Geometry: final body of the model. Coordinates: model frame, mm. A direction names the side the tool comes from. Give positions to 0.01 mm unless a question says otherwise; leave off trailing zeros. Write each loop counter-clockwise with the first axis right and the second up, starting at its lowest first coordinate (ties: lowest second). Pieces come first, ordered by that corner, then holes.
Q1. Cut plane A-A on z = 11. Return the cut outline in (x, y).
Q2. Cut plane D-D on x = 69.5. Return the cut outline in (y, z).
Q3. Draft query along Y for faces 4 (the face through (20, 20, 10)), 5 (the face through (40.46, 0.6, 9.43)), 6 (the face through (12.504, 20.253, 17.395)), 7 (the face through (60, 20, 10)). Return one class per face: pulls with the +Y half, pulls with the -Y half, needs draft (parallel to the pull), parting line crosses it, or undercut.
Q4. Pin query (flat end, axial travel): pin 1 (12 mm diameter, centred on x = 46.5, z = 17, fed in from -Y); pin 2 (1 mm diameter, centred on x = 13, y = 32, fed in from +Z); pin 3 (4 mm diameter, centred on x = 19.5, z = 15.5, fed in from -Y). Return the tip coordinate at first contact, or that it passes through.
Q5. Cut plane B-B on y = 20. Return the cut outline in (x, z), plus the area to 3 significant figures.
Q6. Cut plane C-C on x = 53. Return the cut outline in (y, z).
Q7. Reachability of faces 1 (the face through (40, 15, 18)), 2 (the face through (40, 25, 18)), 3 (the face through (39, 20, 0)) from +Z, -Z, +X, -X, +Y, -Y: full face, straight path, thin tool, end or side. Return the list, or none.
Q8. Line query: L1, parallel to Y at x = 20, z = 20.5; L2, parallel to Z at x = 7.5, y = 37.5; L3, parallel to Y at x = 36, z = 18. Output: solid intervals per line, ascending.
```python
from build123d import *

# Parameters (mm, degrees)
BOSS_EXTRUDE1_DEPTH = 10
FILLET1_R           = 2
FILLET2_R           = 2
SKETCH2_R           = 7.5
BOSS_EXTRUDE3_DEPTH = 15
SKETCH3_R           = 5
CUT_EXTRUDE1_DEPTH  = 15
SKETCH4_R           = 5
CUT_EXTRUDE2_DEPTH  = 15
RIB1_REACH          = 94.871
SKETCH5_WALLS_W     = 202.74175621
SKETCH5_WALLS_H     = 10


with BuildPart() as part:
    # Sketch1 → Boss-Extrude1 (new body)
    with BuildSketch(Plane.XY):
        with BuildLine():
            Line((7, 0), (73, 0))
            ThreePointArc((73, 0), (77.949747468, 2.050252532), (80, 7))
            Line((80, 7), (80, 33))
            ThreePointArc((80, 33), (77.949747468, 37.949747468), (73, 40))
            Line((73, 40), (7, 40))
            ThreePointArc((7, 40), (2.050252532, 37.949747468), (0, 33))
            Line((0, 33), (0, 7))
            ThreePointArc((0, 7), (2.050252532, 2.050252532), (7, 0))
        make_face()
    extrude(amount=BOSS_EXTRUDE1_DEPTH)

    # Fillet1
    fillet1_edges = [part.edges().sort_by_distance(p)[0] for p in [
        (40, 40, 0),
        (2.050252532, 37.949747468, 0),
        (0, 20, 0),
        (2.050252532, 2.050252532, 0),
        (40, 0, 0),
        (77.949747468, 2.050252532, 0),
        (80, 20, 0),
        (77.949747468, 37.949747468, 0),
    ]]
    fillet(fillet1_edges, radius=FILLET1_R)

    # Fillet2
    fillet2_edges = [part.edges().sort_by_distance(p)[0] for p in [
        (2.050252532, 37.949747468, 10),
        (40, 40, 10),
        (77.949747468, 37.949747468, 10),
        (80, 20, 10),
        (77.949747468, 2.050252532, 10),
        (40, 0, 10),
        (2.050252532, 2.050252532, 10),
        (0, 20, 10),
    ]]
    fillet(fillet2_edges, radius=FILLET2_R)

    # Sketch2 → Boss-Extrude3 (add)
    with BuildSketch(Plane.XY.offset(10)):
        with Locations(Location((20, 20, 0), (0, 0, 180))):
            Circle(SKETCH2_R)
        with Locations(Location((60, 20, 0), (0, 0, 180))):
            Circle(SKETCH2_R)
    extrude(amount=BOSS_EXTRUDE3_DEPTH)

    # Sketch3 → Cut-Extrude1 (cut)
    with BuildSketch(Plane.XY.offset(25)):
        with Locations((20, 20)):
            Circle(SKETCH3_R)
    extrude(amount=-CUT_EXTRUDE1_DEPTH, mode=Mode.SUBTRACT)

    # Sketch4 → Cut-Extrude2 (cut)
    with BuildSketch(Plane.XY.offset(25)):
        with Locations((60, 20)):
            Circle(SKETCH4_R)
    extrude(amount=-CUT_EXTRUDE2_DEPTH, mode=Mode.SUBTRACT)

    # Sketch5 walls → Rib1 (add, up to next)
    with BuildSketch(Plane.XY.offset(25), mode=Mode.PRIVATE) as rib1_sk1:
        with Locations((40.936137708, 20)):
            Rectangle(SKETCH5_WALLS_W, SKETCH5_WALLS_H)
    rib1_tool1 = extrude(rib1_sk1.sketch, amount=-RIB1_REACH, mode=Mode.PRIVATE) - part.part
    add(rib1_tool1.solids().sort_by_distance((40.936137708, 20, 25))[0])


solid = part.part
```
Data:
1. outline: (25.59, 15) - (54.41, 15) arc R7.5 ccw (long way) to (54.41, 25) - (25.59, 25) arc R7.5 ccw (long way) to start; hole circle Ø10 at (20, 20); hole circle Ø10 at (60, 20)
2. outline: (0, 2) arc R2 ccw to (2, 0) - (38, 0) arc R2 ccw to (40, 2) - (40, 8) arc R2 ccw to (38, 10) - (2, 10) arc R2 ccw to (0, 8) - close
3. face 4: undercut
3. face 5: pulls with the -Y half
3. face 6: parting line crosses it
3. face 7: undercut
4. pin 1: stops at y = 15
4. pin 2: stops at z = 10
4. pin 3: stops at y = 12.5
5. outline: (0, 2) arc R2 ccw to (2, 0) - (78, 0) arc R2 ccw to (80, 2) - (80, 8) arc R2 ccw to (78, 10) - (67.5, 10) - (67.5, 25) - (65, 25) - (65, 10) - (55, 10) - (55, 25) - (25, 25) - (25, 10) - (15, 10) - (15, 25) - (12.5, 25) - (12.5, 10) - (2, 10) arc R2 ccw to (0, 8) - close
5. area: 1,320 mm2
6. outline: (0, 2) arc R2 ccw to (2, 0) - (38, 0) arc R2 ccw to (40, 2) - (40, 8) arc R2 ccw to (38, 10) - (25, 10) - (25, 25) - (15, 25) - (15, 10) - (2, 10) arc R2 ccw to (0, 8) - close
7. face 1: +Z, -Y
7. face 2: +Z, +Y
7. face 3: -Z, +X, -X, +Y, -Y
8. L1: y = 12.5 to 15, 25 to 27.5
8. L2: z = 0 to 10
8. L3: y = 15 to 25
